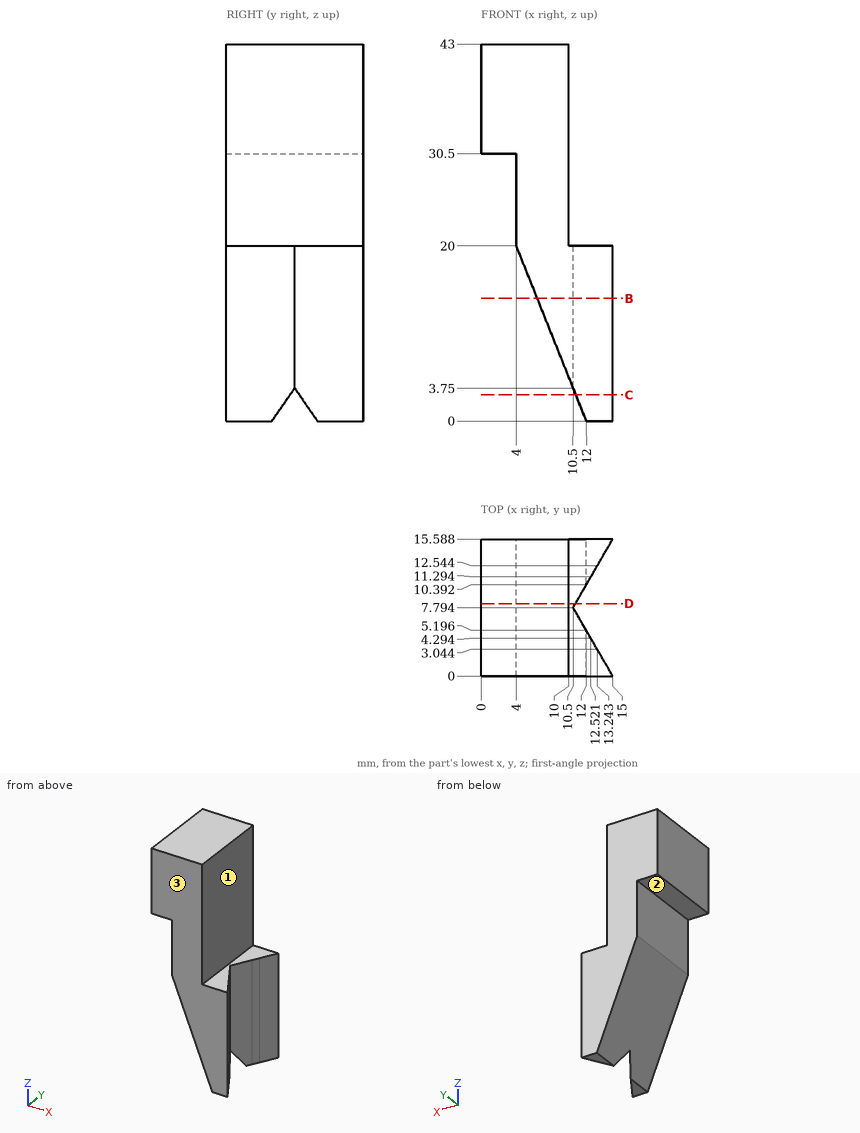
Answer from the drawing. Dimensions are ordinates in mm from the lowest x, y and z of the part. A direction names the side the tool comes from. Coordinates: 2 decimals unless noted, no trailing zeros. Loops run counter-clockwise (first coordinate to the right, second up) from the corner with the lowest first, then second, coordinate; pieces in that order, holes last. Notation, with made-up numbers: (19, 89.5) -> (77, 89.5) arc R11 ccw to (77, 94.5) -> close; hole circle Ø1 at (1.25, 21.25). An arc over 180 degrees is marked (long way). Answer in a Markdown table with one row per item.
Item 1: A cutting plane is placed at D-D on y = 8.25. Determine the outline of the cut face in (x, z).
Returned:
| item | result |
|---|---|
| outline | (0, 30.5) -> (4, 30.5) -> (4, 20) -> (10.76, 3.09) -> (10.76, 20) -> (10, 20) -> (10, 43) -> (0, 43) -> close |
Item 2: A cutting plane is placed at B-B on z = 14. Determine the outline of the cut face in (x, y).
Returned:
| item | result |
|---|---|
| outline | (6.4, 0) -> (15, 0) -> (10.5, 7.79) -> (15, 15.59) -> (6.4, 15.59) -> close |
Item 3: Straight lines are drawn through the part: line 1 along X through (y, z) = (12.25, 25); line 2 along Z through (x, y) = (12.5, 14.25); line 3 along X through (y, z) = (14.5, 33). For each, find the intervals that lie inside material, in ascending order. Write a range as [from, to].
Returned:
| item | result |
|---|---|
| line 1 | x = [4, 10] |
| line 2 | z = [0, 20] |
| line 3 | x = [0, 10] |
Item 4: A cutting plane is placed at C-C on z = 3. Determine the outline of the cut face in (x, y) (1 decimal).
Returned:
| item | result |
|---|---|
| outline | (10.8, 0) -> (15, 0) -> (10.8, 7.3) -> close; (10.8, 8.3) -> (15, 15.6) -> (10.8, 15.6) -> close |
Item 5: Each of these flat-tipped pins is pushed along its axis until it touches: P1, Ø5, axis at y = 3.5, z = 10, coming from the -X side; P2, Ø2.5, axis at x = 12.5, y = 6, coming from the +Z side; P3, Ø3, axis at y = 5, z = 23.5, coming from the -X side; P4, Ø3, axis at x = 5, z = 12, coming from the -Y side. Where does it stop, or does it pass through?
Returned:
| item | result |
|---|---|
| P1 | stops at x = 7 |
| P2 | stops at z = 20 |
| P3 | stops at x = 4 |
| P4 | passes through |
Item 6: For the marked faces 1, 2 and 3, determine the directions among +Z, -Z, +X, -X, +Y, -Y from which every point of the face is accessible in a straight line to the end or side of a thin tool.
Returned:
| item | result |
|---|---|
| face 1 | +Z, +X, +Y, -Y |
| face 2 | -Z, -X, +Y, -Y |
| face 3 | +Z, -Z, +X, -X, -Y |
